from build123d import *

# Parameters (mm, degrees)
F0_W     = 105
F0_H     = 68
F0_R     = 2
F1_DEPTH = 8
F2_R     = 15
F3_DEPTH = 60
F4_W     = 77.2
F4_H     = 77.2
F5_DEPTH = 8
F6_R     = 2.5
F7_DEPTH = 44.4


with BuildPart() as f1:
    # F0 (on Front) → F1 (new body)
    with BuildSketch(Plane.XZ):
        Rectangle(F0_W, F0_H)
        with Locations((-40, -20)):
            Circle(F0_R, mode=Mode.SUBTRACT)
        with Locations((40, -20)):
            Circle(F0_R, mode=Mode.SUBTRACT)
        with Locations((-40, 20)):
            Circle(F0_R, mode=Mode.SUBTRACT)
        with Locations((40, 20)):
            Circle(F0_R, mode=Mode.SUBTRACT)
    extrude(amount=F1_DEPTH)

    # F2 (on Front) → F3 (join)
    with BuildSketch(Plane.XZ):
        Circle(F2_R)
    extrude(amount=-F3_DEPTH)

    # F4 (on face) → F5 (join)
    with BuildSketch(Plane(origin=(0, 60, 0), x_dir=(-1, 0, 0), z_dir=(0, 1, 0))):
        Rectangle(F4_W, F4_H)
    extrude(amount=F5_DEPTH)

    # F6 (on face) → F7 (cut)
    with BuildSketch(Plane(origin=(0, 68, 0), x_dir=(-1, 0, 0), z_dir=(0, 1, 0))):
        with Locations((-19.6, 12.078193)):
            Circle(F6_R)
        with Locations((-19.6, -14.40448)):
            Circle(F6_R)
        with Locations((19.6, -14.40448)):
            Circle(F6_R)
        with Locations((19.6, 12.078193)):
            Circle(F6_R)
    extrude(amount=-F7_DEPTH, mode=Mode.SUBTRACT)


solid = f1.part
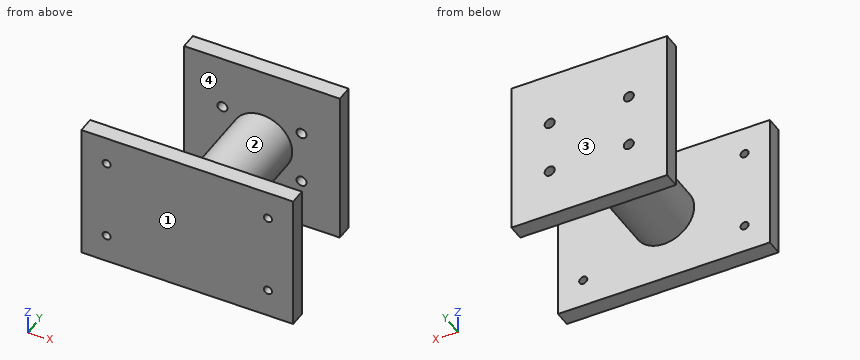
The model under review builds one solid part; all positions refer to its coordinate system, in mm. Face numbers are marked on the shaded views. A direction names the side the tool comes from. Give positions to 0.01 mm unless a question says otherwise; leave off trailing zeros. Order: outer loops, then holes, each group sorted by start corner. A loop starts at its lowest first (then second) coordinate and runs counter-clockwise, first axis right, second up. Notation, with made-up numbers: M 88.25,54 L 132.25,54 A15 cw 132.25,65 Z; hole C 9.5,63.5 d10. An arc over 180 degrees is marked long. One line per question, with ' | ' between items. Start each with the question number.
1) Wall thickness on L1, parallel to Z at x = 19.6, y = 65; L2, parallel to Y at x = 1.5, z = 30; L3, parallel to X at y = -1, z = -19: over which ranges is each line inside the solid? List them lowest first. Write a range as from..to.
2) Consider section D-D, the plane x = -19. Give the boundary of the cut face in (y, z).
3) Clearance check with flat-ended pins moving along their axes: P1, Ø4, axis at x = 19.6, z = 12.08, coming from the +Y side; P2, Ø2, axis at y = 11, z = 8, coming from the +X side; P3, Ø12, axis at y = 49.5, z = 18.5, coming from the +X side. State where each tip first meets the part, or that it passes through.
4) For the marked faces 3 and 4, list the 3-axis set-ups (+Z, -Z, +X, -X, +Y, -Y) from which the entire face can be reached by the end or side of a thin tool; tool diameter is ignored.
5) Consider section C-C, the plane z = -20. Give the boundary of the cut face in (x, y).
6) Consider section B-B, the plane z = 23.5. Give the boundary of the cut face in (x, y), then the cut area to 3 significant figures.
7) Consider section A-A, the plane x = -40. Give the boundary of the cut face in (y, z), then the cut area to 3 significant figures.
8) Mouldability with a two-part tool opening along Z and no side actions: class the marked faces 1 and 2 as pulls with the +Z half, pulls with the -Z half, needs draft (parallel to the pull), parting line crosses it, or undercut.
Found:
1) L1: z = -38.6..-16.9, -11.9..9.58, 14.58..38.6 | L2: y = -8..0, 60..68 | L3: x = -52.5..-41.73, -38.27..38.27, 41.73..52.5
2) outline: M -8,-34 L 0,-34 L 0,34 L -8,34 Z; M 60,-38.6 L 68,-38.6 L 68,-16.83 L 60,-16.83 Z; M 60,-11.98 L 68,-11.98 L 68,9.65 L 60,9.65 Z; M 60,14.51 L 68,14.51 L 68,38.6 L 60,38.6 Z
3) P1: stops at y = 0 | P2: stops at x = 13.27 | P3: stops at x = 8.29
4) face 3: +Z, -Z, +X, -X, +Y | face 4: none
5) outline: M -52.5,-8 L -42,-8 L -42,0 L -52.5,0 Z; M -38.6,60 L 38.6,60 L 38.6,68 L -38.6,68 Z; M -38,-8 L 38,-8 L 38,0 L -38,0 Z; M 42,-8 L 52.5,-8 L 52.5,0 L 42,0 Z
6) outline: M -52.5,-8 L 52.5,-8 L 52.5,0 L -52.5,0 Z; M -38.6,60 L 38.6,60 L 38.6,68 L -38.6,68 Z | area: 1,460 mm²
7) outline: M -8,-34 L 0,-34 L 0,-22 L -8,-22 Z; M -8,-18 L 0,-18 L 0,18 L -8,18 Z; M -8,22 L 0,22 L 0,34 L -8,34 Z | area: 480 mm²
8) face 1: needs draft | face 2: parting line crosses it
